Source: CAD feature listing. Evaluate the final solid. Frame: model axes, mm. Coordinates: 2 decimals unless noted, no trailing zeros. Write each loop counter-clockwise with the first axis right and the second up, starting at its lowest first coordinate (ties: lowest second). Pieces come first, ordered by that corner, then holes. Notation, with made-up numbers: M -28.5,-11.75 L 6.5,-11.75 A22 ccw 6.5,5.25 Z; hole C 78,-16 d2. An arc over 180 degrees is marked long. Write item = value, one per line. Start each with the question number.
1. Section query C-C (y = 11). Output: boundary loops of the cut face in (x, z), then the cut area to 3 significant figures.
2. Pin query (flat end, axial travel): pin 1 Ø5 at (x, y) = (6, 11.5) entering from +Z; pin 2 Ø0.8 at (y, z) = (18, 0.5) entering from +X. Return the tip coordinate at first contact, or that it passes through.
3. Section query D-D (x = -5). Output: boundary loops of the cut face in (y, z), then the cut area to 3 significant figures.
4. Section query A-A (x = 0). Output: boundary loops of the cut face in (y, z), then the cut area to 3 significant figures.
5. Line query: line 1 along X through (y, z) = (21, 0.9); line 2 along Y through (x, z) = (0.5, 0.45); line 3 along Y through (x, z) = (-4, 1.25). Output: solid intervals per line, ascending.
6. Section query B-B (z = 1.15). Output: boundary loops of the cut face in (x, y), then the cut area to 3 significant figures.
```python
from build123d import *

# Parameters (mm, degrees)
SKETCH1_R            = 2.625
BOSS_EXTRUDE1_DEPTH  = 1.5875
FILLET1_R            = 1.778
M4_CLEARANCE_HOLE1_D = 4.5


with BuildPart() as part:
    # Sketch1 → Boss-Extrude1 (new body)
    # profile 1 of 3: a face of its own
    with BuildSketch(Plane.XY):
        with BuildLine():
            ThreePointArc((-14.144818028, 67.686446389), (-1.442639673, 58.098657577), (11.259538681, 67.686446389))
            Line((11.259538681, 67.686446389), (4.907360327, 45.398657577))
            Line((4.907360327, 45.398657577), (4.907360327, -25.721342423))
            Line((4.907360327, -25.721342423), (-7.792639673, -25.721342423))
            Line((-7.792639673, -25.721342423), (-7.792639673, 45.398657577))
            Line((-7.792639673, 45.398657577), (-14.144818028, 67.686446389))
        make_face()
        with Locations((-1.442639673, -19.371342423)):
            Circle(SKETCH1_R, mode=Mode.SUBTRACT)
        with Locations((-1.442639673, 21.268657577)):
            Circle(SKETCH1_R, mode=Mode.SUBTRACT)
    # profile 2 of 3: a face of its own
    with BuildSketch(Plane.XY):
        with Locations((-1.442639673, 21.268657577)):
            Circle(SKETCH1_R)
    # profile 3 of 3: a face of its own
    with BuildSketch(Plane.XY):
        with Locations((-1.442639673, -19.371342423)):
            Circle(SKETCH1_R)
    extrude(amount=BOSS_EXTRUDE1_DEPTH)

    # Fillet1
    fillet1_edges = [part.edges().sort_by_distance(p)[0] for p in [
        (11.259538681, 67.686446389, 0.79375),
        (4.907360327, 45.398657577, 0.79375),
        (4.907360327, -25.721342423, 0.79375),
        (-7.792639673, -25.721342423, 0.79375),
        (-7.792639673, 45.398657577, 0.79375),
        (-14.144818028, 67.686446389, 0.79375),
    ]]
    fillet(fillet1_edges, radius=FILLET1_R)

    # M4 Clearance Hole1 (through all)
    with Locations(Plane.XY.offset(1.5875)):
        with Locations((-1.442639673, -19.371342423), (-1.442639673, 21.268657577)):
            Hole(M4_CLEARANCE_HOLE1_D / 2)


solid = part.part
```
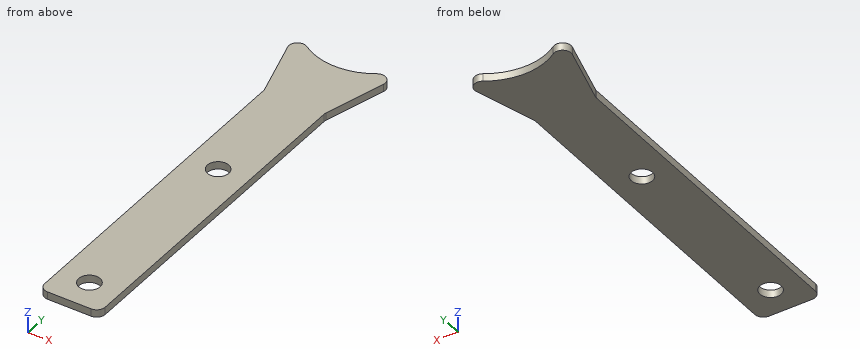
Results are:
q1.outline = M -7.79,0 L 4.91,0 L 4.91,1.59 L -7.79,1.59 Z
q1.area = 20.2 mm^2
q2.pin_1 = 1.59
q2.pin_2 = 4.91
q3.outline = M -25.72,0 L 58.59,0 L 58.59,1.59 L -25.72,1.59 Z
q3.area = 134 mm^2
q4.outline = M -25.72,0 L -21.1,0 L -21.1,1.59 L -25.72,1.59 Z; M -17.64,0 L 19.54,0 L 19.54,1.59 L -17.64,1.59 Z; M 23,0 L 58.18,0 L 58.18,1.59 L 23,1.59 Z
q4.area = 122 mm^2
q5.line_1 = -7.79 to -3.68, 0.79 to 4.91
q5.line_2 = -25.72 to -20.51, -18.24 to 20.13, 22.4 to 58.24
q5.line_3 = -25.72 to 58.35
q6.outline = M -11.49,58.37 L -7.86,45.64 A1.78 cw -7.79,45.15 L -7.79,-23.94 A1.78 ccw -6.01,-25.72 L 3.13,-25.72 A1.78 ccw 4.91,-23.94 L 4.91,45.15 A1.78 cw 4.98,45.64 L 8.6,58.37 A1.78 ccw 5.9,60.33 A13.21 cw -8.79,60.33 A1.78 ccw Z; hole C -1.44,-19.37 d4.5; hole C -1.44,21.27 d4.5
q6.area = 1,100 mm^2
